Print and shaded views of the part. All mm, measured from the part's lowest x, y and z. A direction names the side the tool comes from. Round coordinates to 2 decimals unless told otherwise and drop trailing zeros. Loops run counter-clockwise (first coordinate to the right, second up) from the corner with the lowest first, then second, coordinate; pieces in that order, holes last. Notation, with made-up numbers: (-36.75, 83) - (-9.75, 83) arc R19 cw to (-9.75, 105) - close; hole circle Ø7 at (-28, 86). An arc over 180 degrees is marked (long way). Put each result on its own line as item: value. Start each with the question number.
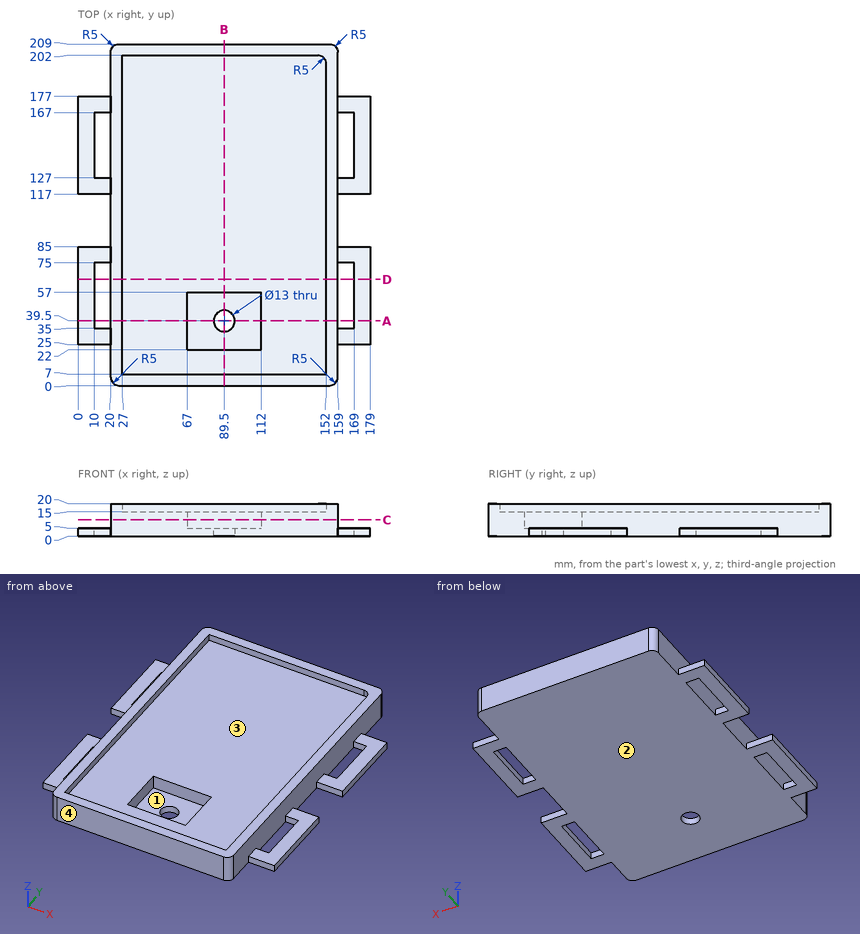
Item 1: Which spindle directions (+Z, -Z, +X, -X, +Y, -Y) get a long thin tool onto all of the face, cutting with end or side? Do the marked faces 1 and 2. Say none if no direction does.
Item 2: Slice it at C-C (z = 10). Give the cut face in (x, y), plus the area to 3 significant figures.
Item 3: Slice it at B-B (x = 89.5). Give the cut face in (y, z), plus the area to 3 significant figures.
Item 4: Slice it at D-D (y = 65). Give the cut face in (x, z).
Item 5: Slice it at A-A (y = 39.5). Give the cut face in (x, z).
Item 6: Drop flat-ended pins along their axis: pin 1 Ø2 at (x, y) = (45.5, 132.5) entering from +Z; pin 2 Ø15 at (x, y) = (89.5, 39.5) entering from +Z; pin 3 Ø6 at (x, z) = (153.5, 18) entering from -Y; pin 4 Ø5 at (y, z) = (42.5, 8.5) entering from -X. Give the stop position or say it passes through.
Item 7: Drill centre lines: probe 1 along Y at (x, z) = (89.5, 2.7); probe 2 along X at (y, z) = (127, 15.25); probe 3 along X at (y, z) = (33, 6.75). Where is each one in solid material? Low to high. Write a range as [from, to].
Item 8: Two-plate mould, pull along X, no slides. Class the marked faces 3 and 4: pulls with the +X half, pulls with the -X half, needs draft (parallel to the pull), parting line crosses it, or undercut.
Computed values:
1. face 1: +Z
1. face 2: -Z, +X, -X, +Y, -Y
2. outline: (20, 5) arc R5 ccw to (25, 0) - (154, 0) arc R5 ccw to (159, 5) - (159, 204) arc R5 ccw to (154, 209) - (25, 209) arc R5 ccw to (20, 204) - close; hole (67, 22) - (112, 22) - (112, 57) - (67, 57) - close
2. area: 27,500 mm^2
3. outline: (0, 0) - (33, 0) - (33, 5) - (22, 5) - (22, 15) - (7, 15) - (7, 20) - (0, 20) - close; (46, 0) - (209, 0) - (209, 20) - (202, 20) - (202, 15) - (57, 15) - (57, 5) - (46, 5) - close
3. area: 2,790 mm^2
4. outline: (0, 0) - (10, 0) - (10, 5) - (0, 5) - close; (20, 0) - (159, 0) - (159, 20) - (152, 20) - (152, 15) - (27, 15) - (27, 20) - (20, 20) - close; (169, 0) - (179, 0) - (179, 5) - (169, 5) - close
5. outline: (0, 0) - (10, 0) - (10, 5) - (0, 5) - close; (20, 0) - (83, 0) - (83, 5) - (67, 5) - (67, 15) - (27, 15) - (27, 20) - (20, 20) - close; (96, 0) - (159, 0) - (159, 20) - (152, 20) - (152, 15) - (112, 15) - (112, 5) - (96, 5) - close; (169, 0) - (179, 0) - (179, 5) - (169, 5) - close
6. pin 1: stops at z = 15
6. pin 2: stops at z = 5
6. pin 3: stops at y = 0
6. pin 4: stops at x = 20
7. probe 1: y = [0, 33], [46, 209]
7. probe 2: x = [20, 27], [152, 159]
7. probe 3: x = [20, 67], [112, 159]
8. face 3: undercut
8. face 4: needs draft
